Can you work these out from the drawing? Everything is in mm from the part's minimum corner. Give positions to 0.01 mm unless a question says otherwise; leave off trailing zeros. Order: outer loops, then holes, each group sorted by start corner. A loop starts at its lowest first (then second) coordinate and runs counter-clockwise, first axis right, second up. Notation, with made-up numbers: (31, -34.5) - (46, -34.5) arc R24 cw to (46, -1.5) - close; hole circle Ø9 at (-13.75, 44). An arc over 180 degrees is marked (long way). Answer as a JSON object with one key per item and string values.
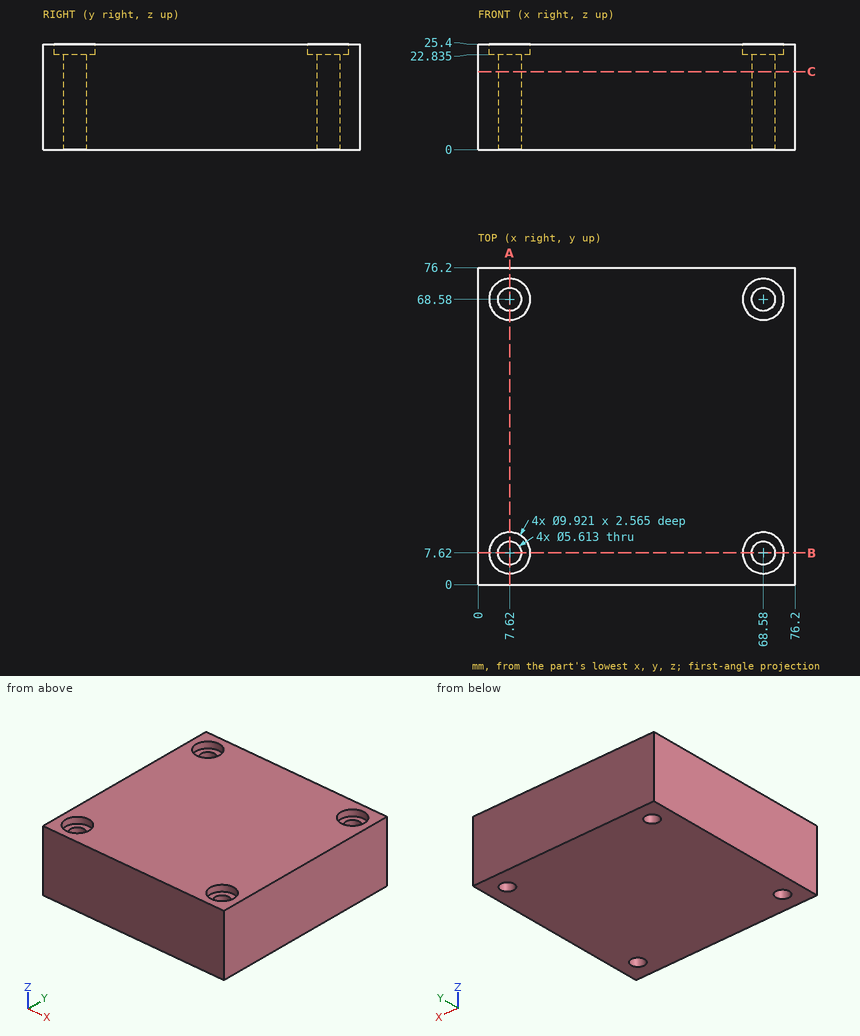
Q1. If we section it at C-C, the plane z = 18.75: Please give me the cut outline in (x, y).
Recorded:
{"outline": "(0, 0) - (76.2, 0) - (76.2, 76.2) - (0, 76.2) - close; hole circle Ø5.61 at (7.62, 7.62); hole circle Ø5.61 at (7.62, 68.58); hole circle Ø5.61 at (68.58, 7.62); hole circle Ø5.61 at (68.58, 68.58)"}
Q2. I need wall thicknesses on L1, parallel to Y at x = 7.62, z = 14.25; L2, parallel to Y at x = 67, z = 23.5. Which ranges of each line are inside material? Lowest first, please.
Recorded:
{"L1": "y = 0 to 4.81, 10.43 to 65.77, 71.39 to 76.2", "L2": "y = 0 to 2.92, 12.32 to 63.88, 73.28 to 76.2"}
Q3. I'm going to push a flat-ended pin straight in: pin 1 Ø6.5 at (x, y) = (68.58, 68.58) entering from +Z (1 decimal). Where does the tip first touch, or does it pass through?
Recorded:
{"pin 1": "stops at z = 22.8"}
Q4. If we section it at A-A, the plane x = 7.62: Please give me the cut outline in (y, z) (1 decimal), then the cut area to 3 significant figures.
Recorded:
{"outline": "(0, 0) - (4.8, 0) - (4.8, 22.8) - (2.7, 22.8) - (2.7, 25.4) - (0, 25.4) - close; (10.4, 0) - (65.8, 0) - (65.8, 22.8) - (63.6, 22.8) - (63.6, 25.4) - (12.6, 25.4) - (12.6, 22.8) - (10.4, 22.8) - close; (71.4, 0) - (76.2, 0) - (76.2, 25.4) - (73.5, 25.4) - (73.5, 22.8) - (71.4, 22.8) - close", "area": "1,630 mm^2"}
